Autodesk Inventor part; units mm, degrees
ref_plane "YZ Plane" through (0, 0, 0) normal (1, 0, 0) x (0, 1, 0)
ref_plane "XZ Plane" through (0, 0, 0) normal (0, 1, 0) x (-1, 0, 0)
ref_plane "XY Plane" through (0, 0, 0) normal (0, 0, 1) x (1, 0, 0)
sketch "Sketch1" plane through (0, 0, 0) normal (0, 1, 0) x (-1, 0, 0)
  line L0 (-61.2, -88.9) -> (61.2, -88.9)
  line L1 (76.2, -73.9) -> (76.2, 58.9)
  line L2 (46.2, 88.9) -> (-46.2, 88.9)
  line L3 (-76.2, 58.9) -> (-76.2, -73.9)
  line L4 (-76.2, -88.9) -> (76.2, 88.9) construction
  line L5 (76.2, -88.9) -> (-76.2, 88.9) construction
  arc A0 (76.2, 58.9) -> (46.2, 88.9) centre (46.2, 58.9) ccw
  arc A1 (-46.2, 88.9) -> (-76.2, 58.9) centre (-46.2, 58.9) ccw
  arc A2 (61.2, -88.9) -> (76.2, -73.9) centre (61.2, -73.9) ccw
  arc A3 (-76.2, -73.9) -> (-61.2, -88.9) centre (-61.2, -73.9) ccw
  circle A4 centre (0, 73.025) radius 7.9375
  circle A5 centre (0, 0) radius 27.5
  dimension "d0" = 177.8
  dimension "d1" = 152.4
  dimension "d2" = 30
  dimension "d3" = 15
  dimension "d4" = 15.875
  dimension "d5" = 15.875
  dimension "d9" = 55
extrude "Extrusion1" add sketch "Sketch1" along normal blind 26.75
fillet "Fillet1" radius 4 8 edges at (71.8066, 26.75, -84.5066) (0, 26.75, -88.9) (-71.8066, 26.75, -84.5066) (-76.2, 26.75, -7.5) (-67.4132, 26.75, 80.1132) (0, 26.75, 88.9) (67.4132, 26.75, 80.1132) (76.2, 26.75, -7.5)
properties part number "Durometer_Base"
Geometry check sheet. Reference: the model listing, model coordinates, mm. Round coordinates to 2 decimals unless told otherwise and drop trailing zeros. Loops run counter-clockwise (first coordinate to the right, second up) from the corner with the lowest first, then second, coordinate; pieces in that order, holes last. Notation, with made-up numbers: (-3.75, 69.25) -> (28.25, 69.25) arc R21 cw to (28.25, 77.25) -> close; hole circle Ø8 at (-2.75, 38). An arc over 180 degrees is marked (long way). Answer as a JSON object with one key per item and string values. Group by question number.
Item 1: Thickness scan on line 1 along Z through (x, y) = (0, 12.5); line 2 along X through (y, z) = (24, 79); line 3 along Z through (x, y) = (-25, 18.75). Record the ranges inside material, lowest first.
Item 2: Release check for a two-part mould opening along Z. For faces 1 (the face through (-1, 11, 88.9)), 2 (the face through (1, 11, -88.9)), 3 (the face through (1.721, 13.188, 80.774)) record: pulls with the +Z half, pulls with the -Z half, needs draft (parallel to the pull), parting line crosses it, or undercut.
Item 3: Depth check by flat-ended pin: pin 1 Ø12 at (x, y) = (-52.5, 5.5) entering from +Z; pin 2 Ø2 at (x, y) = (50.5, 7.5) entering from +Z. Enter the tip coordinate at first touch or a pass-through.
Item 4: Cross-section at B-B, the plane x = 0. Record the cut outline in (y, z), plus the area to 3 significant figures.
Item 5: Cross-section at C-C, the plane x = 19.5. Record the cut outline in (y, z).
Item 6: Cross-section at A-A, the plane z = 0. Record the cut outline in (x, y).
Item 7: Cross-section at D-D, the plane y = 4.25. Record the cut outline in (x, z) (1 decimal).
Determined:
{
 "1": {"line 1": "z = -88.9 to -27.5, 27.5 to 65.09, 80.96 to 88.9", "line 2": "x = -68.2 to -5.23, 5.23 to 68.2", "line 3": "z = -88.9 to -11.46, 11.46 to 88.9"},
 "2": {"face 1": "pulls with the +Z half", "face 2": "pulls with the -Z half", "face 3": "undercut"},
 "3": {"pin 1": "stops at z = 88.9", "pin 2": "stops at z = 88.72"},
 "4": {"outline": "(0, -88.9) -> (22.75, -88.9) arc R4 ccw to (26.75, -84.9) -> (26.75, -27.5) -> (0, -27.5) -> close; (0, 27.5) -> (26.75, 27.5) -> (26.75, 65.09) -> (0, 65.09) -> close; (0, 80.96) -> (26.75, 80.96) -> (26.75, 84.9) arc R4 ccw to (22.75, 88.9) -> (0, 88.9) -> close", "area": "2,850 mm²"},
 "5": {"outline": "(0, -88.9) -> (22.75, -88.9) arc R4 ccw to (26.75, -84.9) -> (26.75, -19.39) -> (0, -19.39) -> close; (0, 19.39) -> (26.75, 19.39) -> (26.75, 84.9) arc R4 ccw to (22.75, 88.9) -> (0, 88.9) -> close"},
 "6": {"outline": "(-76.2, 0) -> (-27.5, 0) -> (-27.5, 26.75) -> (-72.2, 26.75) arc R4 ccw to (-76.2, 22.75) -> close; (27.5, 0) -> (76.2, 0) -> (76.2, 22.75) arc R4 ccw to (72.2, 26.75) -> (27.5, 26.75) -> close"},
 "7": {"outline": "(-76.2, -73.9) arc R15 ccw to (-61.2, -88.9) -> (61.2, -88.9) arc R15 ccw to (76.2, -73.9) -> (76.2, 58.9) arc R30 ccw to (46.2, 88.9) -> (-46.2, 88.9) arc R30 ccw to (-76.2, 58.9) -> close; hole circle Ø55 at (0, 0); hole circle Ø15.9 at (0, 73)"}
}
